Part model, mm, in its own coordinate system. Face numbers are marked on the shaded views. A direction names the side the tool comes from. Round coordinates to 2 decimals unless told otherwise and drop trailing zeros. Order: outer loops, then holes, each group sorted by start corner. A loop starts at its lowest first (then second) coordinate and runs counter-clockwise, first axis right, second up. Notation, with made-up numbers: M 30.5,76.5 L 66.5,76.5 A23 cw 66.5,94.5 Z; hole C 15,70.25 d1. An arc over 180 degrees is marked long. One line per question, with ' | ' between items.
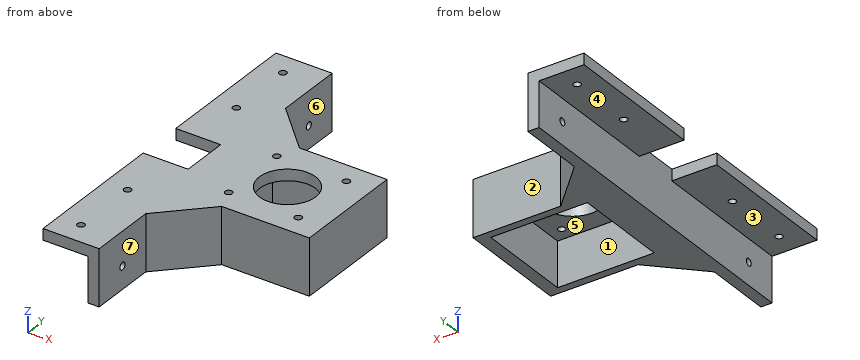
from build123d import *

# Parameters (mm, degrees)
F0_W      = 150
F0_H      = 25
F1_DEPTH  = 5
F2_W      = 50
F2_H      = 25
F3_DEPTH  = 59
F4_W      = 43
F4_H      = 43
F5_DEPTH  = 20
F7_D      = 3.2
F7_DEPTH  = 8
F7_TIP    = 0.9613769904
F6_R      = 12.5
F8_DEPTH  = 5.001
F10_D     = 3.2
F10_DEPTH = 8
F10_TIP   = 0.9613769904
F11_SIZE  = 20
F12_W     = 150
F12_H     = 5
F13_DEPTH = 20
F14_W     = 21
F14_H     = 5
F15_DEPTH = 20
F17_D     = 3.2
F17_DEPTH = 8
F17_TIP   = 0.9613769904


with BuildPart() as f1:
    # F0 (on Right) → F1 (new body)
    with BuildSketch(Plane.YZ):
        with Locations((75, 12.5)):
            Rectangle(F0_W, F0_H)
    extrude(amount=F1_DEPTH)

    # F2 (on face) → F3 (join)
    with BuildSketch(Plane.YZ.offset(5)):
        with Locations((75, 12.5)):
            Rectangle(F2_W, F2_H)
    extrude(amount=F3_DEPTH)

    # F4 (on face) → F5 (cut)
    with BuildSketch(Plane(origin=(0, 0, 0), x_dir=(1, 0, 0), z_dir=(0, 0, -1))):
        with Locations((37, -75)):
            Rectangle(F4_W, F4_H)
    extrude(amount=-F5_DEPTH, mode=Mode.SUBTRACT)

    # F7
    with Locations(Plane(origin=(0, 0, 20), x_dir=(1, 0, 0), z_dir=(0, 0, -1))):
        with Locations((21.5, -59.5), (52.5, -59.5), (52.5, -90.5), (21.5, -90.5)):
            Hole(F7_D / 2, depth=F7_DEPTH)
            with Locations((0, 0, -(F7_DEPTH + F7_TIP / 2))):  # 118° drill point
                Cone(0, F7_D / 2, F7_TIP, mode=Mode.SUBTRACT)

    # F6 (on face) → F8 (cut, through all)
    with BuildSketch(Plane(origin=(0, 0, 20), x_dir=(1, 0, 0), z_dir=(0, 0, -1))):
        with Locations((37, -75)):
            Circle(F6_R)
    extrude(amount=-F8_DEPTH, mode=Mode.SUBTRACT)

    # F10
    with Locations(Plane.YZ.offset(5)):
        with Locations((15, 10), (135, 10)):
            Hole(F10_D / 2, depth=F10_DEPTH)
            with Locations((0, 0, -(F10_DEPTH + F10_TIP / 2))):  # 118° drill point
                Cone(0, F10_D / 2, F10_TIP, mode=Mode.SUBTRACT)

    # F11
    f11_edges = [f1.edges().sort_by_distance(p)[0] for p in [
        (5, 50, 12.5),
        (5, 100, 12.5),
    ]]
    chamfer(f11_edges, length=F11_SIZE)

    # F12 (on face) → F13 (join)
    with BuildSketch(Plane(origin=(0, 0, 0), x_dir=(0, -1, 0), z_dir=(-1, 0, 0))):
        with Locations((-75, 22.5)):
            Rectangle(F12_W, F12_H)
    extrude(amount=F13_DEPTH)

    # F14 (on face) → F15 (cut, through all)
    with BuildSketch(Plane(origin=(-20, 0, 0), x_dir=(0, -1, 0), z_dir=(-1, 0, 0))):
        with Locations((-75, 22.5)):
            Rectangle(F14_W, F14_H)
    extrude(amount=-F15_DEPTH, mode=Mode.SUBTRACT)

    # F17
    with Locations(Plane.XY.offset(25)):
        with Locations((-10, 10), (-10, 40), (-10, 110), (-10, 140)):
            Hole(F17_D / 2, depth=F17_DEPTH)
            with Locations((0, 0, -(F17_DEPTH + F17_TIP / 2))):  # 118° drill point
                Cone(0, F17_D / 2, F17_TIP, mode=Mode.SUBTRACT)


solid = f1.part
1) Probe line 1 (X direction, y = 59.5, z = 23.55); line 2 (X direction, y = 75, z = 23.1); line 3 (X direction, y = 57.5, z = 14.25). List the from-to ranges inside material, lowest first. Write a range as [from, to].
The answers:
line 1: x = [-20, 19.9], [23.1, 50.9], [54.1, 64] | line 2: x = [0, 24.5], [49.5, 64] | line 3: x = [0, 15.5], [58.5, 64]
2) Drop flat-ended pins along their axis: pin 1 (4 mm diameter, centred on y = 107, z = 13.5, fed in from -X); pin 2 (12 mm diameter, centred on x = 15.5, z = 8, fed in from +Y); pin 3 (10 mm diameter, centred on x = -11.5, y = 21, fed in from -Z). Give the stop position or say it passes through.
The answers:
pin 1: stops at x = 0 | pin 2: stops at y = 115.5 | pin 3: stops at z = 20
3) Two-plate mould, pull along Y, no slides. Class the marked faces 1, 2 and 3: released by +Y, released by -Y, zero draft, split by the parting line, or undercut.
The answers:
face 1: undercut | face 2: released by +Y | face 3: zero draft
4) Saw through at D-D (x = -10). List the corners of the cut face in (y, z), plus the area to 3 significant figures.
The answers:
outline: M 0,20 L 8.4,20 L 8.4,25 L 0,25 Z; M 11.6,20 L 38.4,20 L 38.4,25 L 11.6,25 Z; M 41.6,20 L 64.5,20 L 64.5,25 L 41.6,25 Z; M 85.5,20 L 108.4,20 L 108.4,25 L 85.5,25 Z; M 111.6,20 L 138.4,20 L 138.4,25 L 111.6,25 Z; M 141.6,20 L 150,20 L 150,25 L 141.6,25 Z | area: 581 mm²
5) Saw through at A-A (z = 10). List the corners of the cut face in (x, y).
The answers:
outline: M 0,0 L 5,0 L 5,13.4 L 0,13.4 Z; M 0,16.6 L 5,16.6 L 5,30 L 25,50 L 64,50 L 64,100 L 25,100 L 5,120 L 5,133.4 L 0,133.4 Z; M 0,136.6 L 5,136.6 L 5,150 L 0,150 Z; hole M 15.5,53.5 L 58.5,53.5 L 58.5,96.5 L 15.5,96.5 Z
6) Saw through at B-B (x = 37). List the corners of the cut face in (y, z), plus the area to 3 significant figures.
The answers:
outline: M 50,0 L 53.5,0 L 53.5,20 L 62.5,20 L 62.5,25 L 50,25 Z; M 87.5,20 L 96.5,20 L 96.5,0 L 100,0 L 100,25 L 87.5,25 Z | area: 265 mm²
7) Saw through at C-C (y = 40). List the corners of the cut face in (x, z), plus the area to 3 significant figures.
The answers:
outline: M -20,20 L -11.6,20 L -11.6,25 L -20,25 Z; M -8.4,20 L 0,20 L 0,0 L 15,0 L 15,25 L -8.4,25 Z | area: 459 mm²
8) Which spindle directions (+Z, -Z, +X, -X, +Y, -Y) get a long thin tool onto all of the face, cutting with end or side? Do the marked faces 4, 5, 6 and 7. Say none if no direction does.
The answers:
face 4: -Z, -X, +Y, -Y | face 5: -Z | face 6: +Z, -Z, +X, +Y | face 7: +Z, -Z, +X, -Y
